For this review, take the finished solid that the model builds, in its own axes (mm). A direction names the side the tool comes from. Give positions to 0.01 mm unless a question says otherwise; leave off trailing zeros. Order: outer loops, then holes, each group sorted by start corner. A loop starts at its lowest first (then second) coordinate and runs counter-clockwise, first axis right, second up.
Item 1: Consider section C-C (x = -15). Give the boundary of the cut face in (y, z).
Item 2: Machinability: for faces 1 (the flat face through (-11.2, 5.842, -40.3)), 2 (the cylindrical face through (38.839, 2.88, 25.412)), which of the approach directions +Z, -Z, +X, -X, +Y, -Y give a long, thin tool a straight path to every point of the face, cutting with its end or side? Answer none if there is none.
Item 3: Consider section B-B (z = 0). Give the boundary of the cut face in (x, y).
Item 4: For P1, Ø4, axis at x = -17.5, z = 39.5, coming from the +Y side; P2, Ø12, axis at x = 3.5, y = 27, coming from the -Z side; P3, Ø8.5, axis at x = -23.11, z = 40.03, coming from the +Y side; P4, Ø5, axis at y = 23.5, z = 8, coming from the -X side, all flat-tipped, find the tip position at first contact; note any pin that passes through.
Item 5: The part is to be moulded in two halves that separate along Z. For faces 3 (the cylindrical face through (-22.818, 15.453, -29.759)), 4 (the flat face through (36.2, 0, 11.2)), 5 (the cylindrical face through (-40.417, 18.333, -8.975)), say which applies: released by +Z, released by -Z, zero draft, split by the parting line, or undercut.
Item 6: For probe 1 along X at (y, z) = (2.05, 0); probe 2 along X at (y, z) = (5, 40.5); probe 3 along X at (y, z) = (25, -7), list the stretches that pass through material, from the lowest coordinate up.
Item 7: Consider section A-A (x = 0). Give the boundary of the cut face in (y, z), plus the area to 3 significant figures.
Item 8: Consider section D-D (y = 2). Give the number of separate pieces and of enclosed holes in the cut face, plus the area to 3 significant figures.
```python
from build123d import *

# Parameters (mm, degrees)
SKETCH4_R                  = 49.2125
BOSS_EXTRUDE2_DEPTH        = 30.48
SKETCH5_OUTSIDE_W          = 128.922
SKETCH5_OUTSIDE_H          = 128.922
SKETCH5_OUTSIDE_R          = 41.402
CUT_EXTRUDE3_DEPTH         = 24.638
SKETCH6_R                  = 37.5
CUT_EXTRUDE4_DEPTH         = 76.978751717
F_6_0_204_DIAMETER_HOLE2_D = 5.1816
CIRPATTERN5_COUNT          = 12


with BuildPart() as part:
    # Sketch4 → Boss-Extrude2 (new body)
    with BuildSketch(Plane(origin=(0, 0, 0), x_dir=(1, 0, 0), z_dir=(0, 1, 0))):
        with Locations(Location((0, 0, 0), (0, 0, 90))):
            Circle(SKETCH4_R)
    extrude(amount=BOSS_EXTRUDE2_DEPTH)

    # Sketch5 outside → Cut-Extrude3 (cut)
    with BuildSketch(Plane(origin=(0, 30.48, 0), x_dir=(1, 0, 0), z_dir=(0, 1, 0))):
        Rectangle(SKETCH5_OUTSIDE_W, SKETCH5_OUTSIDE_H)
        with Locations(Location((0, 0, 0), (0, 0, 270))):
            Circle(SKETCH5_OUTSIDE_R, mode=Mode.SUBTRACT)
    extrude(amount=-CUT_EXTRUDE3_DEPTH, mode=Mode.SUBTRACT)

    # Sketch6 → Cut-Extrude4 (cut, through all)
    with BuildSketch(Plane(origin=(0, 30.48, 0), x_dir=(1, 0, 0), z_dir=(0, 1, 0))):
        with Locations(Location((0, 0, 0), (0, 0, 270))):
            Circle(SKETCH6_R)
    extrude(amount=-CUT_EXTRUDE4_DEPTH, mode=Mode.SUBTRACT)

    # #6 (0.204) Diameter Hole2 (through all)
    with Locations(Plane(origin=(0, 5.842, 0), x_dir=(1, 0, 0), z_dir=(0, 1, 0))):
        with Locations((0, 46.228)):
            f_6_0_204_diameter_hole2 = Hole(F_6_0_204_DIAMETER_HOLE2_D / 2)

    # CirPattern5: #6 (0.204) Diameter Hole2 ×12 about axis
    cirpattern5_axis = Axis((0, 0, 0), (0, 1, 0))
    for i in range(1, CIRPATTERN5_COUNT):
        add(f_6_0_204_diameter_hole2.rotate(cirpattern5_axis, i * 360 / CIRPATTERN5_COUNT), mode=Mode.SUBTRACT)


solid = part.part
```
Resolved:
1. outline: (0, -46.87) - (5.84, -46.87) - (5.84, -38.59) - (30.48, -38.59) - (30.48, -34.37) - (0, -34.37) - close; (0, 34.37) - (30.48, 34.37) - (30.48, 38.59) - (5.84, 38.59) - (5.84, 46.87) - (0, 46.87) - close
2. face 1: +Y
2. face 2: +Y, -Y
3. outline: (-49.21, 0) - (-48.82, 0) - (-48.82, 5.84) - (-49.21, 5.84) - close; (-43.64, 0) - (-37.5, 0) - (-37.5, 30.48) - (-41.4, 30.48) - (-41.4, 5.84) - (-43.64, 5.84) - close; (37.5, 0) - (43.64, 0) - (43.64, 5.84) - (41.4, 5.84) - (41.4, 30.48) - (37.5, 30.48) - close; (48.82, 0) - (49.21, 0) - (49.21, 5.84) - (48.82, 5.84) - close
4. P1: stops at y = 30.48
4. P2: stops at z = -41.4
4. P3: stops at y = 5.84
4. P4: stops at x = -41.04
5. face 3: undercut
5. face 4: zero draft
5. face 5: split by the parting line
6. probe 1: x = -49.21 to -48.82, -43.64 to -37.5, 37.5 to 43.64, 48.82 to 49.21
6. probe 2: x = -27.96 to -25.66, -20.57 to 20.57, 25.66 to 27.96
6. probe 3: x = -40.81 to -36.84, 36.84 to 40.81
7. outline: (0, -49.21) - (5.84, -49.21) - (5.84, -48.82) - (0, -48.82) - close; (0, -43.64) - (5.84, -43.64) - (5.84, -41.4) - (30.48, -41.4) - (30.48, -37.5) - (0, -37.5) - close; (0, 37.5) - (30.48, 37.5) - (30.48, 41.4) - (5.84, 41.4) - (5.84, 43.64) - (0, 43.64) - close; (0, 48.82) - (5.84, 48.82) - (5.84, 49.21) - (0, 49.21) - close
7. area: 269 mm2
8. separate pieces: 1
8. enclosed holes: 13
8. area: 2,940 mm2
